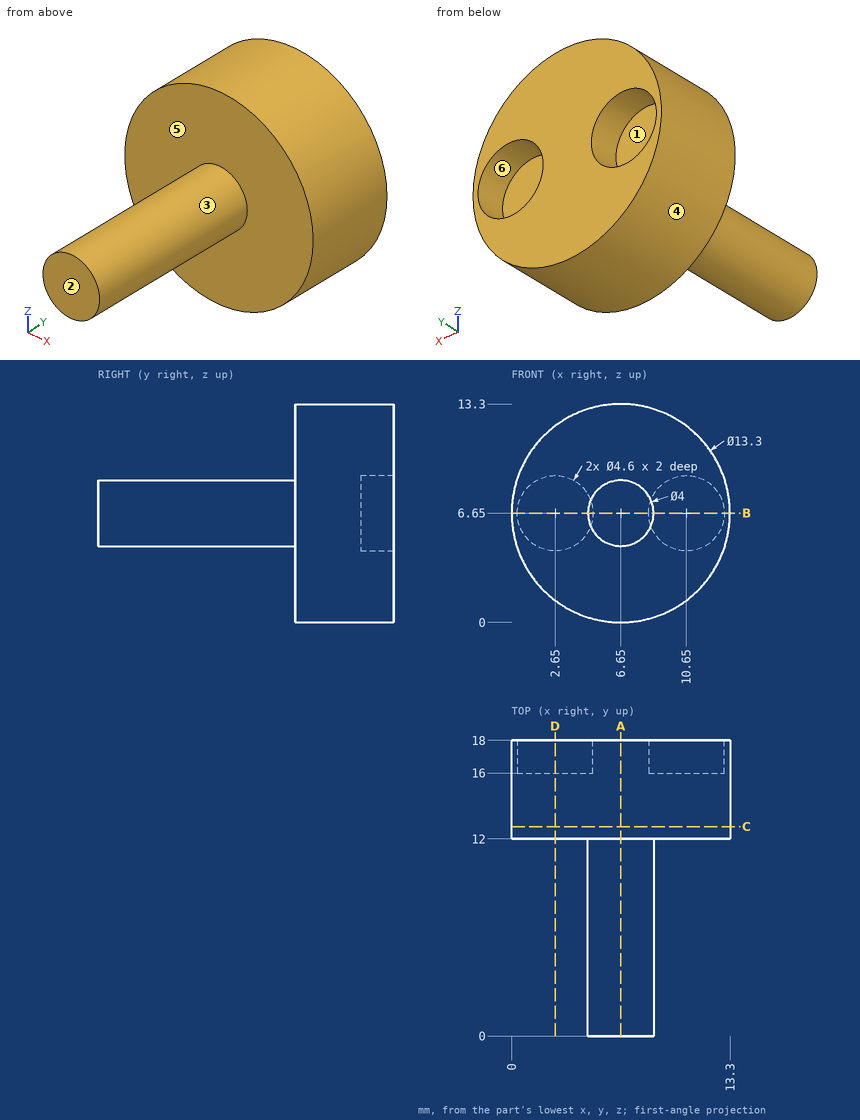
Here's the drawing with two shaded views (mm, measured from the low corner). I have some questions. A direction names the side the tool comes from. Round coordinates to 2 decimals unless told otherwise and drop trailing zeros. Loops run counter-clockwise (first coordinate to the right, second up) from the corner with the lowest first, then second, coordinate; pieces in that order, holes last. Notation, with made-up numbers: (7, -19.5) - (16, -19.5) arc R17 ccw to (16, -6.5) - close; hole circle Ø2 at (59.5, 69). An arc over 180 degrees is marked (long way). Use CSV: the item, a comma, the result in double quotes. Start each with the question number.
1) If we section it at C-C on y = 12.75: Write out the boundary of the cut face in (x, z), plus the area to 3 significant figures.
2) If we section it at D-D on x = 2.65: Write out the boundary of the cut face in (y, z), plus the area to 3 significant figures.
3) For pin 1 Ø3 at (y, z) = (4, 4) entering from -X; pin 2 Ø1 at (y, z) = (13, 5) entering from +X; pin 3 Ø5 at (x, y) = (4.5, 14.5) entering from -Z; pin 4 Ø2 at (y, z) = (13.5, 5) entering from -X, each with a flat end and sliding along its axis, tell me the tip position at first contact or that it passes through.
4) We'd pull the mould along X, two halves only. Please class the marked faces 4, 5 and 6: released by +X, released by -X, zero draft, split by the parting line, or undercut.
5) If we section it at B-B on z = 6.65: Write out the boundary of the cut face in (x, y).
6) Please list where these lines run through material, in increasing order: probe 1 along Y at (x, z) = (4.5, 4.25); probe 2 along Y at (x, z) = (10.5, 7.25); probe 3 along Z at (x, y) = (10.65, 16.8). Write a range as [from, to].
7) If we section it at A-A on x = 6.65: Write out the boundary of the cut face in (y, z), plus the area to 3 significant figures.
8) For the marked faces 1, 2 and 3, which set-ups out of +Z, -Z, +X, -X, +Y, -Y let a thin tool reach every point of the face, with its end or its side?
Geometry results:
1,outline,"circle Ø13.3 at (6.65, 6.65)"
1,area,"139 mm2"
2,outline,"(12, 1.34) - (18, 1.34) - (18, 4.35) - (16, 4.35) - (16, 8.95) - (18, 8.95) - (18, 11.96) - (12, 11.96) - close"
2,area,"54.5 mm2"
3,pin 1,"stops at x = 5.01"
3,pin 2,"stops at x = 13.2"
3,pin 3,"stops at z = 0"
3,pin 4,"stops at x = 0.03"
4,face 4,"split by the parting line"
4,face 5,"zero draft"
4,face 6,"undercut"
5,outline,"(0, 12) - (4.65, 12) - (4.65, 0) - (8.65, 0) - (8.65, 12) - (13.3, 12) - (13.3, 18) - (12.95, 18) - (12.95, 16) - (8.35, 16) - (8.35, 18) - (4.95, 18) - (4.95, 16) - (0.35, 16) - (0.35, 18) - (0, 18) - close"
6,probe 1,"y = [12, 18]"
6,probe 2,"y = [12, 16]"
6,probe 3,"z = [1.34, 4.35], [8.95, 11.96]"
7,outline,"(0, 4.65) - (12, 4.65) - (12, 0) - (18, 0) - (18, 13.3) - (12, 13.3) - (12, 8.65) - (0, 8.65) - close"
7,area,"128 mm2"
8,face 1,"+Y"
8,face 2,"+Z, -Z, +X, -X, -Y"
8,face 3,"-Y"
